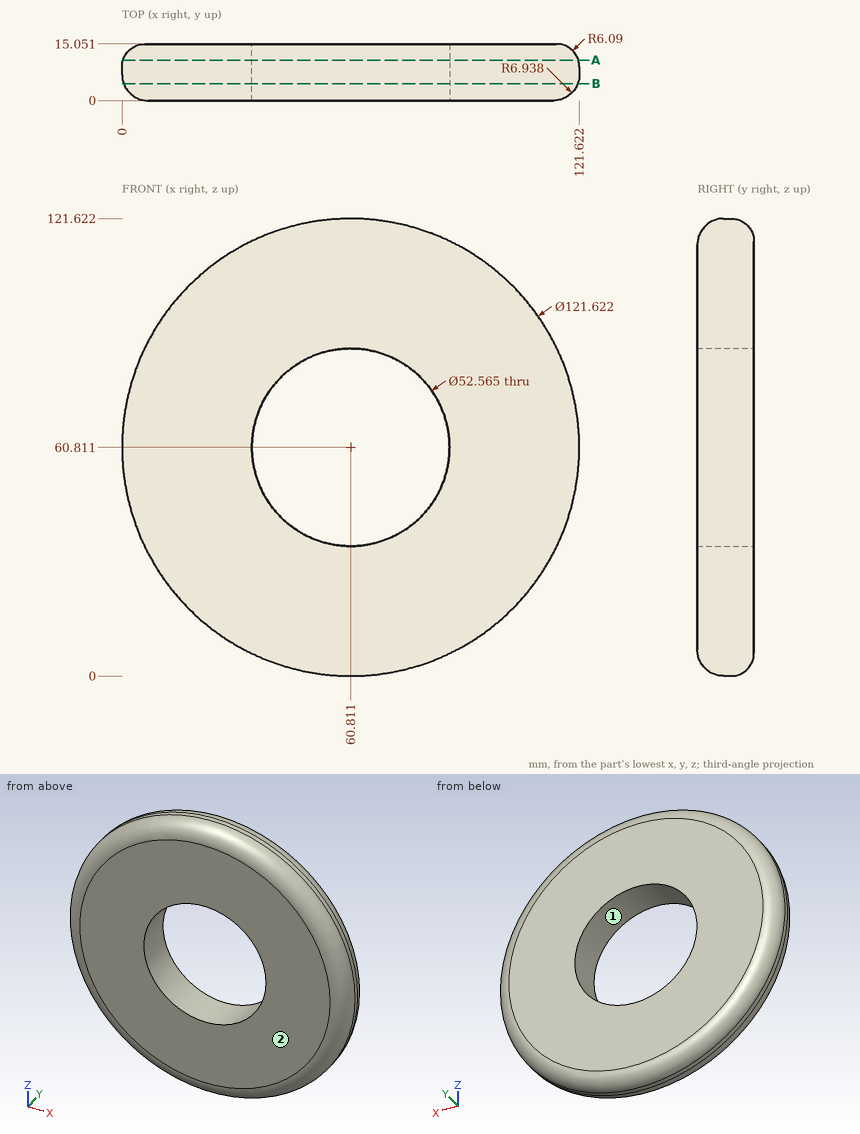
Can you work these out from the drawing? Everything is in mm from the part's minimum corner. Coordinates: 2 decimals unless noted, no trailing zeros. Order: outer loops, then holes, each group sorted by start corner. A loop starts at its lowest first (then second) coordinate and runs counter-clockwise, first axis right, second up. Notation, with made-up numbers: M 82,71 L 100,71 A14 cw 100,76 Z; hole C 31,29.5 d11. An arc over 180 degrees is marked long. Answer as CSV lines item,"result". Start each with the question number.
1. I want a section at B-B, the plane y = 4.5. Write out the boundary of the cut face in (x, z) (1 decimal).
2. We'd pull the mould along X, two halves only. Please class the marked faces 1 and 2: released by +X, released by -X, zero draft, split by the parting line, or undercut.
3. For pin 1 (5 mm diameter, centred on x = 15, z = 98, fed in from -Y); pin 2 (2 mm diameter, centred on x = 32, y = 3, fed in from +Z); pin 3 (5 mm diameter, centred on x = 27.5, y = 2.5, fed in from +Z) (1 decimal), each with a flat end and sliding along its axis, tell me the tip position at first contact or that it passes through.
4. I want a section at A-A, the plane y = 10.75. Write out the boundary of the cut face in (x, z) (1 decimal).
5. I need wall thicknesses on line 1 (Z direction, x = 85, y = 14) (1 decimal); line 2 (Z direction, x = 82.5, y = 9.25) (1 decimal); line 3 (X direction, y = 9.75, z = 53.5) (1 decimal). Which ranges of each line are inside material? Lowest first, please. Write a range as [from, to].
Recorded:
1,outline,"C 60.8,60.8 d120.7; hole C 60.8,60.8 d52.6"
2,face 1,"undercut"
2,face 2,"zero draft"
3,pin 1,"stops at y = 0.52"
3,pin 2,"stops at z = 113.84"
3,pin 3,"stops at z = 112.2"
4,outline,"C 60.8,60.8 d121.1; hole C 60.8,60.8 d52.6"
5,line 1,"z = [7.9, 50.5], [71.1, 113.7]"
5,line 2,"z = [4, 46], [75.7, 117.6]"
5,line 3,"x = [0.5, 35.6], [86.1, 121.1]"
